Drawing for the job (mm, zero at the part's lowest x, y, z). Give positions to 0.01 mm unless a question says otherwise; leave off trailing zeros. Loops run counter-clockwise (first coordinate to the right, second up) from the corner with the lowest first, then second, coordinate; pieces in that order, holes last. Notation, with made-up numbers: M -27,-36.5 L -5,-36.5 A27 cw -5,-0.5 Z; hole C 60.25,74 d3. An arc over 180 degrees is marked long. Use CSV: the item, a comma, the result in double quotes. Start each with the question number.
(1) Wall check: line 1 along Z through (x, y) = (52, 53); line 2 along Y through (x, z) = (35.5, 18.25); line 3 along X through (y, z) = (23, 25.75). Give the ranges that are in metal, low to high. Write a range as from..to.
(2) Slice it at C-C on y = 37.5. List the corners of the cut face in (x, z).
(3) Two-plate mould, pull along Y, no slides. Class the marked faces 1, 2 and 3: pulls with the +Y half, pulls with the -Y half, needs draft (parallel to the pull), parting line crosses it, or undercut.
(4) Slice it at B-B on x = 50. List the corners of the cut face in (y, z).
(5) Slice it at A-A on z = 22.75. List the corners of the cut face in (x, y).
(6) Flat gauge pins, fed straight in: P1, Ø6, axis at y = 51.5, z = 19.5, coming from the +X side; P2, Ø1, axis at x = 76, y = 18.5, coming from the -Z side. Where does each tip first touch, or does it go through?
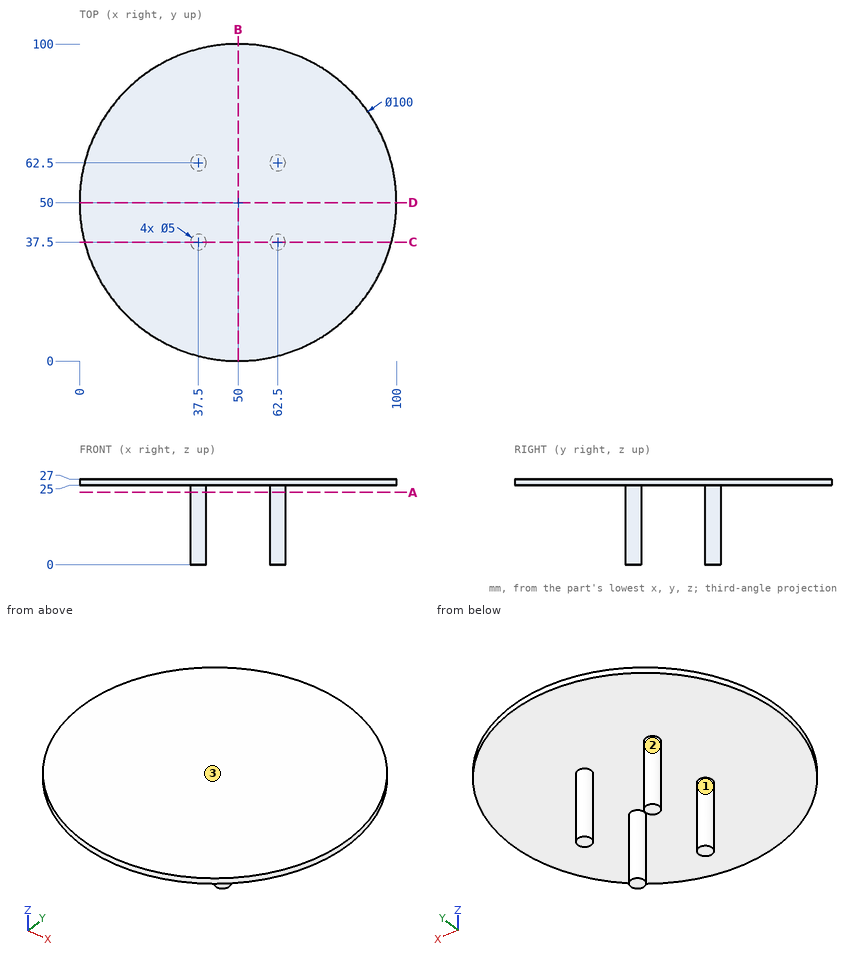
Reply:
1,line 1,"z = 25..27"
1,line 2,"y = 36..39, 61..64"
1,line 3,"x = 7.92..92.08"
2,outline,"M 1.59,25 L 35,25 L 35,0 L 40,0 L 40,25 L 60,25 L 60,0 L 65,0 L 65,25 L 98.41,25 L 98.41,27 L 1.59,27 Z"
3,face 1,"undercut"
3,face 2,"undercut"
3,face 3,"needs draft"
4,outline,"M 0,25 L 100,25 L 100,27 L 0,27 Z"
5,outline,"C 37.5,37.5 d5; C 37.5,62.5 d5; C 62.5,37.5 d5; C 62.5,62.5 d5"
6,P1,"passes through"
6,P2,"stops at z = 25"
